Check sheet for the modelled part. Datum: model origin and axes. Units: mm. Round coordinates to 2 decimals unless told otherwise and drop trailing zeros. Order: outer loops, then holes, each group sorted by start corner. A loop starts at its lowest first (then second) coordinate and runs counter-clockwise, first axis right, second up. Notation, with made-up numbers: (-39, 77) -> (20, 77) arc R11 ccw to (20, 84) -> close; hole circle Ø4 at (69.5, -33). An arc over 180 degrees is marked (long way). Use CSV: the item, a comma, the result in double quotes.
```python
from build123d import *

# Parameters (mm, degrees)
F0_R      = 23.1993727041
F1_DEPTH  = 12.7
F2_R      = 23.1993727041
F3_DEPTH  = 12.7
F6_DEPTH  = 6.35
F7_DEPTH  = 6.35
F8_SIZE   = 6.34999
F9_SIZE   = 6.34999
F10_DEPTH = 25.4
F11_DEPTH = 127


# Not quite as in the source:
# - a fillet or chamfer is up to 0.001 mm smaller than in the source, because OpenCascade refuses the exact size


with BuildPart() as f1:
    # F0 (on Front) → F1 (new body)
    with BuildSketch(Plane.XZ):
        with Locations((-16.9251933694, -16.9251933694)):
            Circle(F0_R)
    extrude(amount=F1_DEPTH)

    # F2 (on face) → F3 (join)
    with BuildSketch(Plane(origin=(0, 0, 0), x_dir=(-1, 0, 0), z_dir=(0, 1, 0))):
        with Locations((16.9251933694, -16.9251933694)):
            Circle(F2_R)
    extrude(amount=F3_DEPTH)

    # F4 (on face) → F6 (join)
    with BuildSketch(Plane(origin=(0, 12.7, 0), x_dir=(-1, 0, 0), z_dir=(0, 1, 0))):
        Polygon((34.987336153, -18.3641740003), (16.5690030176, 1.1906780042), (-1.1369494142, -15.4862127385), (17.2813837212, -35.041064743), align=None)
    extrude(amount=F6_DEPTH)

    # F5 (on face) → F7 (join)
    with BuildSketch(Plane.XZ.offset(12.7)):
        Polygon((1.1413726115, -15.5428544637), (-16.5892601531, 1.1910649658), (-34.9917593503, -18.3075322751), (-17.2611265857, -35.0414517045), align=None)
    extrude(amount=F7_DEPTH)

    # F8 (size 6.35 in the source; OpenCascade refuses exactly that, so slightly less here)
    f8_edges = [f1.edges().sort_by_distance(p)[0] for p in [
        (-8.072217, 19.05, -25.263639),
        (-26.13436, 19.05, -26.702619),
        (-25.77817, 19.05, -8.586748),
        (-7.716027, 19.05, -7.147767),
    ]]
    chamfer(f8_edges, length=F8_SIZE)

    # F9 (size 6.35 in the source; OpenCascade refuses exactly that, so slightly less here)
    f9_edges = [f1.edges().sort_by_distance(p)[0] for p in [
        (-8.059877, -19.05, -25.292153),
        (-7.723944, -19.05, -7.175895),
        (-25.79051, -19.05, -8.558234),
        (-26.126443, -19.05, -26.674492),
    ]]
    chamfer(f9_edges, length=F9_SIZE)

    # F10 (cut): faces of the model
    f10_faces = [f1.faces().sort_by_distance(p)[0] for p in [
        (-39.4683887232, -12.7, -16.9251933694),
        (-39.4683887232, -12.7, -16.9251933694),
        (-39.4683887232, -12.7, -16.9251933694),
        (-39.4683887232, -12.7, -16.9251933694),
    ]]
    extrude(f10_faces, amount=-F10_DEPTH, mode=Mode.SUBTRACT)

    # F11 (cut): faces of the model
    f11_faces = [f1.faces().sort_by_distance(p)[0] for p in [
        (-6.6175325, 12.7, -23.7415572289),
        (-27.2328542388, 12.7, -10.1088295099),
    ]]
    extrude(f11_faces, amount=-F11_DEPTH, mode=Mode.SUBTRACT)


solid = f1.part
```
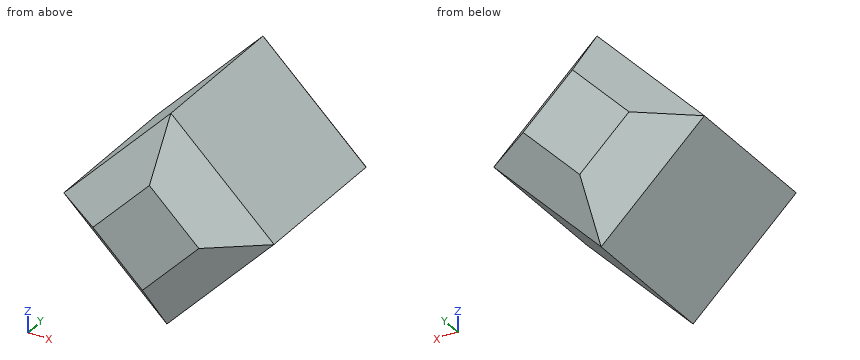
Q1. Go/stop test with flat-tipped pins: pin 1 (5 mm diameter, centred on y = -10, z = -12.5, fed in from +X); pin 2 (5 mm diameter, centred on x = -29.5, y = -6.5, fed in from -Z); pin 3 (3 mm diameter, centred on x = -5.5, y = -0.5, fed in from -Z); pin 4 (18.5 mm diameter, centred on x = -8.5, z = -10, fed in from -Y). Record where each tip stops, or that it passes through.
Result sheet:
pin 1,"stops at x = 0.57"
pin 2,"stops at z = -25.85"
pin 3,"stops at z = -24.13"
pin 4,"stops at y = -19.05"
Q2. Sectioned sample at C-C, the plane y = 11. Enter the section's corners in (x, z), then the cut area to 3 significant figures.
Result sheet:
outline,"(-34.96, -18.34) -> (-17.27, -35.03) -> (1.11, -15.51) -> (-16.58, 1.18) -> close"
area,"652 mm^2"
Q3. Scan lines: L1, parallel to X at y = 14.5, z = -13.5; L2, parallel to Y at x = -20, z = -30; L3, parallel to X at y = 13.5, z = -6. Record each from-to range of solid material in increasing order.
Result sheet:
L1,"x = -27.93 to -3.6"
L2,"y = -14.49 to 14.51"
L3,"x = -22.24 to -10.1"
